Can you work these out from the model? Positions are in its coordinate system, mm. Face numbers are marked on the shaded views. A direction names the side the tool comes from. Round coordinates to 2 decimals unless told otherwise and drop trailing zeros. Order: outer loops, then holes, each group sorted by start corner. A loop starts at its lowest first (then second) coordinate and runs counter-clockwise, first axis right, second up.
Q1. If we section it at D-D (y = 19.5): Please give me the cut outline in (x, z), plus the area to 3 significant figures.
Q2. If I drill on line 1 (Y direction, x = 55.3, z = -52.5); line 2 (X direction, y = 4, z = -22.5); line 3 (Z direction, x = 29.5, y = 4.25), over which ranges is the centre line in solid material (lowest first)?
Q3. For the marked faces 1 and 2, which set-ups out of +Z, -Z, +X, -X, +Y, -Y let a thin tool reach every point of the face, with its end or its side?
Q4. We'd pull the mould along X, two halves only. Please class the marked faces 3, 4 and 5: pulls with the +X half, pulls with the -X half, needs draft (parallel to the pull), parting line crosses it, or undercut.
Q5. If we section it at A-A (z = -11.5): Please give me the cut outline in (x, y), plus the area to 3 significant figures.
Q6. If we section it at B-B (x = 35): Please give me the cut outline in (y, z), plus the area to 3 significant figures.
Q7. Will these pins go through, and if not, where does the flat tip stop? P1, Ø2, axis at x = 43.5, y = 15, coming from the -Z side; P2, Ø3.5, axis at y = 19.5, z = -52.5, coming from the -X side; P3, Ø10, axis at x = 48.5, y = 11.5, coming from the -Z side.
Q8. If we section it at C-C (z = -45.5): Please give me the cut outline in (x, y).
from build123d import *

# Parameters (mm, degrees)
SALIENTE_EXTRUIR2_DEPTH = 25
CROQUIS2_R              = 4
CROQUIS2_R_2            = 1.5
CORTAR_EXTRUIR1_DEPTH   = 10
CROQUIS3_R              = 4
CROQUIS3_R_2            = 1.5
CORTAR_EXTRUIR2_DEPTH   = 60


with BuildPart() as part:
    # Croquis1 → Saliente-Extruir2 (new body)
    with BuildSketch(Plane(origin=(0, 0, 0), x_dir=(1, 0, 0), z_dir=(0, 1, 0))):
        with BuildLine():
            Line((0, 1.84), (0, 65))
            Line((0, 65), (2, 65))
            Line((2, 65), (2, 3))
            ThreePointArc((2, 3), (2.292893219, 2.292893219), (3, 2))
            Line((3, 2), (53, 2))
            ThreePointArc((53, 2), (53.707106781, 2.292893219), (54, 3))
            Line((54, 3), (54, 65))
            Line((54, 65), (56, 65))
            Line((56, 65), (56, 1.84))
            ThreePointArc((56, 1.84), (55.461076477, 0.538923523), (54.16, 0))
            Line((54.16, 0), (1.84, 0))
            ThreePointArc((1.84, 0), (0.538923523, 0.538923523), (0, 1.84))
        make_face()
    extrude(amount=SALIENTE_EXTRUIR2_DEPTH)

    # Croquis2 → Cortar-Extruir1 (cut)
    with BuildSketch(Plane.XY):
        with Locations((28, 12.5)):
            Circle(CROQUIS2_R)
        with Locations((28, 19.5)):
            Circle(CROQUIS2_R_2)
        with Locations((28, 5.5)):
            Circle(CROQUIS2_R_2)
        with Locations((35, 12.5)):
            Circle(CROQUIS2_R_2)
        with Locations((21, 12.5)):
            Circle(CROQUIS2_R_2)
    extrude(amount=-CORTAR_EXTRUIR1_DEPTH, mode=Mode.SUBTRACT)

    # Croquis3 → Cortar-Extruir2 (cut)
    with BuildSketch(Plane(origin=(56, 0, 0), x_dir=(0, 0, -1), z_dir=(1, 0, 0))):
        with BuildLine():
            Line((65, 25), (52.5, 25))
            ThreePointArc((52.5, 25), (61.338834765, 21.338834765), (65, 12.5))
            Line((65, 12.5), (65, 25))
        make_face()
        with BuildLine():
            Line((65, 0), (65, 12.5))
            ThreePointArc((65, 12.5), (61.338834765, 3.661165235), (52.5, 0))
            Line((52.5, 0), (65, 0))
        make_face()
        with Locations((52.5, 12.5)):
            Circle(CROQUIS3_R)
        with Locations((45.5, 12.5)):
            Circle(CROQUIS3_R_2)
        with Locations((52.5, 19.5)):
            Circle(CROQUIS3_R_2)
        with Locations((59.5, 12.5)):
            Circle(CROQUIS3_R_2)
        with Locations((52.5, 5.5)):
            Circle(CROQUIS3_R_2)
    extrude(amount=-CORTAR_EXTRUIR2_DEPTH, mode=Mode.SUBTRACT)


solid = part.part
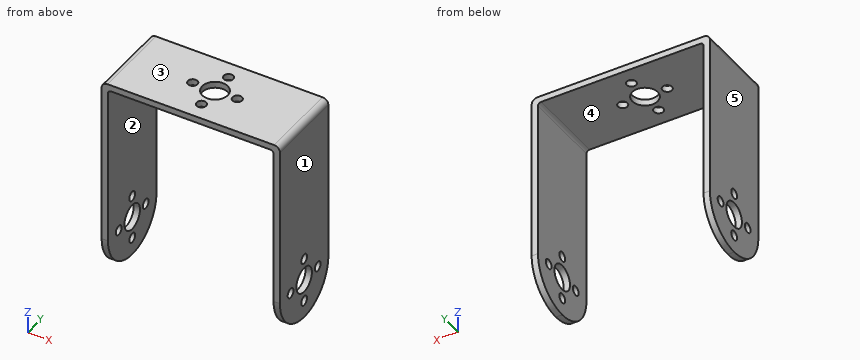
Solution:
1. outline: (0, -62.86) - (2, -62.86) - (2, -54) - (0, -54) - close; (0, -51) - (2, -51) - (2, -3) arc R1 cw to (3, -2) - (26.5, -2) - (26.5, 0) - (1.84, 0) arc R1.84 ccw to (0, -1.84) - close; (29.5, -2) - (53, -2) arc R1 cw to (54, -3) - (54, -51) - (56, -51) - (56, -1.84) arc R1.84 ccw to (54.16, 0) - (29.5, 0) - close; (54, -62.86) - (56, -62.86) - (56, -54) - (54, -54) - close
1. area: 336 mm2
2. line 1: y = 0 to 4, 7 to 8.5, 16.5 to 18, 21 to 25
2. line 2: x = 0 to 2, 54 to 56
2. line 3: z = -2 to 0
3. face 1: +Z, -Z, +X, +Y, -Y
3. face 2: -Z, +Y, -Y
4. face 3: needs draft
4. face 4: undercut
4. face 5: pulls with the -X half
5. outline: (0, 0) - (2, 0) - (2, 25) - (0, 25) - close; (54, 0) - (56, 0) - (56, 25) - (54, 25) - close
5. area: 100 mm2
6. outline: (0, -2) - (11, -2) - (11, 0) - (0, 0) - close; (14, -2) - (25, -2) - (25, 0) - (14, 0) - close
6. area: 44.0 mm2
7. P1: stops at z = -2
7. P2: stops at x = 0
7. P3: stops at z = -2.13
8. outline: (0, 0) - (2, 0) - (2, 11) - (0, 11) - close; (0, 14) - (2, 14) - (2, 25) - (0, 25) - close; (54, 0) - (56, 0) - (56, 11) - (54, 11) - close; (54, 14) - (56, 14) - (56, 25) - (54, 25) - close
